The model under review builds one solid part; all positions refer to its coordinate system, in mm. Coordinates: 2 decimals unless noted, no trailing zeros. Order: outer loops, then holes, each group sorted by start corner. A loop starts at its lowest first (then second) coordinate and runs counter-clockwise, first axis right, second up. Notation, with made-up numbers: M 3,-37 L 18,-37 A25 ccw 18,-15 Z; hole C 71,78 d5. An arc over 180 degrees is marked long. Write each question's results on one line, items separated by ' | '.
from build123d import *

# Parameters (mm, degrees)
SKETCH2_W           = 60
SKETCH2_H           = 35.5
BOSS_EXTRUDE1_DEPTH = 3
SKETCH3_W           = 3
SKETCH3_H           = 10
BOSS_EXTRUDE2_DEPTH = 3
SKETCH4_W           = 20
SKETCH4_H           = 3
CUT_EXTRUDE2_DEPTH  = 3
SKETCH5_W           = 20
SKETCH5_H           = 6.5
CUT_EXTRUDE3_DEPTH  = 10


with BuildPart() as part:
    # Sketch2 → Boss-Extrude1 (new body)
    with BuildSketch(Plane(origin=(0, 0, 0), x_dir=(1, 0, 0), z_dir=(0, 1, 0))):
        Rectangle(SKETCH2_W, SKETCH2_H)
    extrude(amount=BOSS_EXTRUDE1_DEPTH)

    # Sketch3 → Boss-Extrude2 (add)
    with BuildSketch(Plane(origin=(0, 0, 0), x_dir=(1, 0, 0), z_dir=(0, 1, 0))):
        with Locations((-31.5, 2.5)):
            Rectangle(SKETCH3_W, SKETCH3_H)
        with Locations((31.5, 2.5)):
            Rectangle(SKETCH3_W, SKETCH3_H)
    extrude(amount=BOSS_EXTRUDE2_DEPTH)

    # Sketch4 → Cut-Extrude2 (cut)
    with BuildSketch(Plane(origin=(0, 3, 0), x_dir=(1, 0, 0), z_dir=(0, 1, 0))):
        with Locations((-20, 16.25)):
            Rectangle(SKETCH4_W, SKETCH4_H)
        with Locations((20, 16.25)):
            Rectangle(SKETCH4_W, SKETCH4_H)
    extrude(amount=-CUT_EXTRUDE2_DEPTH, mode=Mode.SUBTRACT)

    # Sketch5 → Cut-Extrude3 (cut)
    with BuildSketch(Plane(origin=(0, 3, 0), x_dir=(1, 0, 0), z_dir=(0, 1, 0))):
        with Locations((0, -14.5)):
            Rectangle(SKETCH5_W, SKETCH5_H)
    extrude(amount=-CUT_EXTRUDE3_DEPTH, mode=Mode.SUBTRACT)


solid = part.part
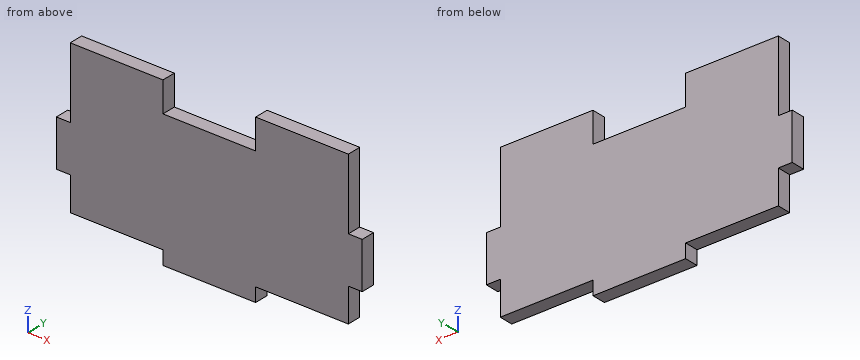
1) For pin 1 (1.5 mm diameter, centred on y = 1.5, z = -12.5, fed in from +X); pin 2 (1.5 mm diameter, centred on x = 32, y = 1.5, fed in from -Z); pin 3 (1.5 mm diameter, centred on x = -31.5, y = 1, fed in from +Z); pin 4 (3 mm diameter, centred on x = -12, z = -10, fed in from -Y), all flat-tipped, find the tip position at first contact; note any pin that passes through.
Solutions:
pin 1: x = 30 | pin 2: z = -7.5 | pin 3: z = 2.5 | pin 4: y = 0
2) Take a section at C-C on x = -28.5. State the section outline as (y, z) points.
Solutions:
outline: M 0,-14.75 L 3,-14.75 L 3,17.75 L 0,17.75 Z
3) Take a section at D-D on z = -9. State the section outline as (x, y) points.
Solutions:
outline: M -30,0 L 30,0 L 30,3 L -30,3 Z
4) To check wall thickness, follow line 1 along X through (y, z) = (2.4, 15); line 2 along Z through (x, y) = (-5.5, 0.4); line 3 along X through (y, z) = (1.85, -10). State the ranges of each line that lie inside material, in increasing order.
Solutions:
line 1: -30 to -10, 10 to 30 | line 2: -17.75 to 11.25 | line 3: -30 to 30
5) Take a section at B-B on y = 2.35. State the section outline as (x, z) points.
Solutions:
outline: M -33,-7.5 L -30,-7.5 L -30,-14.75 L -10,-14.75 L -10,-17.75 L 10,-17.75 L 10,-14.75 L 30,-14.75 L 30,-7.5 L 33,-7.5 L 33,2.5 L 30,2.5 L 30,17.75 L 10,17.75 L 10,11.25 L -10,11.25 L -10,17.75 L -30,17.75 L -30,2.5 L -33,2.5 Z
6) Take a section at A-A on z = 13. State the section outline as (x, y) points, plus the area to 3 significant figures.
Solutions:
outline: M -30,0 L -10,0 L -10,3 L -30,3 Z; M 10,0 L 30,0 L 30,3 L 10,3 Z | area: 120 mm2
